from build123d import *

# Parameters (mm, degrees)
SKETCH2_R               = 60
BOSS_EXTRUDE1_DEPTH     = 20
SKETCH3_W               = 60
SKETCH3_H               = 25
CUT_EXTRUDE1_DEPTH      = 8
CUT_EXTRUDE2_DEPTH      = 40
CUT_EXTRUDE2_DEPTH_BACK = 17
SKETCH4_R               = 6
SKETCH5_R               = 16
CUT_EXTRUDE3_DEPTH      = 16.25
SKETCH6_R               = 4
CUT_EXTRUDE4_DEPTH      = 88.177978871
CUT_EXTRUDE5_DEPTH      = 88.177978871


with BuildPart() as part:
    # Sketch2 → Boss-Extrude1 (new body)
    with BuildSketch(Plane(origin=(0, 0, 0), x_dir=(1, 0, 0), z_dir=(0, 1, 0))):
        with Locations(Location((0, 0, 0), (0, 0, 270))):
            Circle(SKETCH2_R)
    extrude(amount=BOSS_EXTRUDE1_DEPTH)

    # Sketch3 → Cut-Extrude1 (cut)
    with BuildSketch(Plane.XZ):
        Rectangle(SKETCH3_W, SKETCH3_H)
    extrude(amount=-CUT_EXTRUDE1_DEPTH, mode=Mode.SUBTRACT)

    # Sketch4 → Cut-Extrude2 (cut, two sides: drawn at the far end of the back side and taken through both)
    with BuildSketch(Plane.XY.offset(-12.5).offset(-CUT_EXTRUDE2_DEPTH_BACK)):
        with Locations((-17.5, 0)):
            Circle(SKETCH4_R)
        with Locations((17.5, 0)):
            Circle(SKETCH4_R)
    extrude(amount=CUT_EXTRUDE2_DEPTH + CUT_EXTRUDE2_DEPTH_BACK, mode=Mode.SUBTRACT)

    # Sketch5 → Cut-Extrude3 (cut, symmetric)
    with BuildSketch(Plane.XY):
        with Locations((-17.5, 0)):
            Circle(SKETCH5_R)
        with Locations((17.5, 0)):
            Circle(SKETCH5_R)
    extrude(amount=CUT_EXTRUDE3_DEPTH, both=True, mode=Mode.SUBTRACT)

    # Sketch6 → Cut-Extrude4 (cut, through all)
    with BuildSketch(Plane(origin=(0, 20, 0), x_dir=(1, 0, 0), z_dir=(0, 1, 0))):
        with Locations(Location((0, 40, 0), (0, 0, 270))):
            Circle(SKETCH6_R)
        with Locations(Location((40, 0, 0), (0, 0, 270))):
            Circle(SKETCH6_R)
        with Locations(Location((0, -40, 0), (0, 0, 270))):
            Circle(SKETCH6_R)
        with Locations(Location((-40, 0, 0), (0, 0, 270))):
            Circle(SKETCH6_R)
    extrude(amount=-CUT_EXTRUDE4_DEPTH, mode=Mode.SUBTRACT)

    # Sketch7 → Cut-Extrude5 (cut, through all)
    with BuildSketch(Plane(origin=(0, 20, 0), x_dir=(1, 0, 0), z_dir=(0, 1, 0))):
        with BuildLine():
            Line((-35, 27.5), (35, 27.5))
            ThreePointArc((35, 27.5), (40, 22.5), (35, 17.5))
            Line((35, 17.5), (-35, 17.5))
            ThreePointArc((-35, 17.5), (-40, 22.5), (-35, 27.5))
        make_face()
        with BuildLine():
            Line((-35, -27.5), (35, -27.5))
            ThreePointArc((35, -27.5), (40, -22.5), (35, -17.5))
            Line((35, -17.5), (-35, -17.5))
            ThreePointArc((-35, -17.5), (-40, -22.5), (-35, -27.5))
        make_face()
    extrude(amount=-CUT_EXTRUDE5_DEPTH, mode=Mode.SUBTRACT)


solid = part.part
Work out the finished part from the listing and answer in its coordinate system (mm). A direction names the side the tool comes from. Coordinates: 2 decimals unless noted, no trailing zeros. Write each loop counter-clockwise with the first axis right and the second up, starting at its lowest first coordinate (ties: lowest second). Pieces come first, ordered by that corner, then holes.
1. The part is cut by section B-B, the plane z = -40. Write down the section's boundary in (x, y).
Results list:
outline: (-44.72, 0) - (-4, 0) - (-4, 20) - (-44.72, 20) - close; (4, 0) - (44.72, 0) - (44.72, 20) - (4, 20) - close
2. For faces 5 (the cylindrical face through (40, 10.1, 22.6)), 6 (the cylindrical face through (17.6, 6, -28.5)), 7 (the flat face through (0, 0, 16)), determine the directions among +Z, -Z, +X, -X, +Y, -Y from which every point of the face is accessible in a straight line to the end or side of a thin tool.
Results list:
face 5: +Y, -Y
face 6: -Y
face 7: +Z, -Z, +X, -X, -Y
3. For a pull along Z with two mould halves and no side action, classify faces 1 (the flat face through (0, 5, -12.5)), 2 (the cylindrical face through (2.64, 9.86, -59.94)), 3 (the flat face through (17, 8, 16.25)), 4 (the flat face through (0, 0, -16)) as +Z half, -Z half, draft (parallel to the pull), parting line (faces both ways), or undercut.
Results list:
face 1: undercut
face 2: parting line
face 3: undercut
face 4: draft
4. The part is cut by section A-A, the plane x = 0. Write down the section's boundary in (y, z).
Results list:
outline: (0, -60) - (20, -60) - (20, -44) - (0, -44) - close; (0, -36) - (20, -36) - (20, -27.5) - (0, -27.5) - close; (0, -17.5) - (20, -17.5) - (20, 17.5) - (0, 17.5) - (0, 12.5) - (8, 12.5) - (8, -12.5) - (0, -12.5) - close; (0, 27.5) - (20, 27.5) - (20, 36) - (0, 36) - close; (0, 44) - (20, 44) - (20, 60) - (0, 60) - close
5. Flat-ended cylindrical pins translate along their axes: pin 1 (2 mm diameter, centred on x = 1.5, y = 2.5, fed in from +Z); pin 2 (6 mm diameter, centred on x = -4.5, y = 5.5, fed in from -Z); pin 3 (1.8 mm diameter, centred on x = -20, y = 4, fed in from +Z); pin 4 (6.5 mm diameter, centred on x = -40, z = 0, fed in from -Y). Find the tip coordinate at first contact, or state that the pin passes through.
Results list:
pin 1: stops at z = 60
pin 2: stops at z = -59.98
pin 3: stops at z = 56.88
pin 4: passes through
6. Consider line 1 along X through (y, z) = (11.75, 0); line 2 along X through (y, z) = (13.75, 0); line 3 along Z through (x, y) = (30, 3.5). Determine where each line is inside the solid, lowest interval first.
Results list:
line 1: x = -60 to -44, -36 to -28.36, -6.64 to 6.64, 28.36 to 36, 44 to 60
line 2: x = -60 to -44, -36 to -25.68, -9.32 to 9.32, 25.68 to 36, 44 to 60
line 3: z = -51.96 to -27.5, -17.5 to -16.25, 16.25 to 17.5, 27.5 to 51.96
7. The part is cut by section C-C, the plane y = 11. State how many separate pieces and enclosed holes the cut face has, and give its area (3 significant figures).
Results list:
separate pieces: 1
enclosed holes: 8
area: 8,040 mm2
8. The part is cut by section D-D, the plane y = 18.5. Write down the section's boundary in (x, z).
Results list:
outline: circle Ø120 at (0, 0); hole circle Ø8 at (-40, 0); hole (-35, -27.5) - (35, -27.5) arc R5 ccw to (35, -17.5) - (-35, -17.5) arc R5 ccw to start; hole (-35, 17.5) - (35, 17.5) arc R5 ccw to (35, 27.5) - (-35, 27.5) arc R5 ccw to start; hole circle Ø8 at (0, -40); hole circle Ø8 at (0, 40); hole circle Ø8 at (40, 0)
